Print and shaded views of the part. All mm, measured from the part's lowest x, y and z. A direction names the side the tool comes from. Round coordinates to 2 decimals unless told otherwise and drop trailing zeros. Loops run counter-clockwise (first coordinate to the right, second up) from the corner with the lowest first, then second, coordinate; pieces in that order, holes last. Notation, with made-up numbers: (-4.5, -31.75) - (25.5, -31.75) arc R16 ccw to (25.5, -18.75) - close; hole circle Ø5 at (-34.5, 20). An arc over 180 degrees is marked (long way). Answer as a JSON object with one key per item and string values.
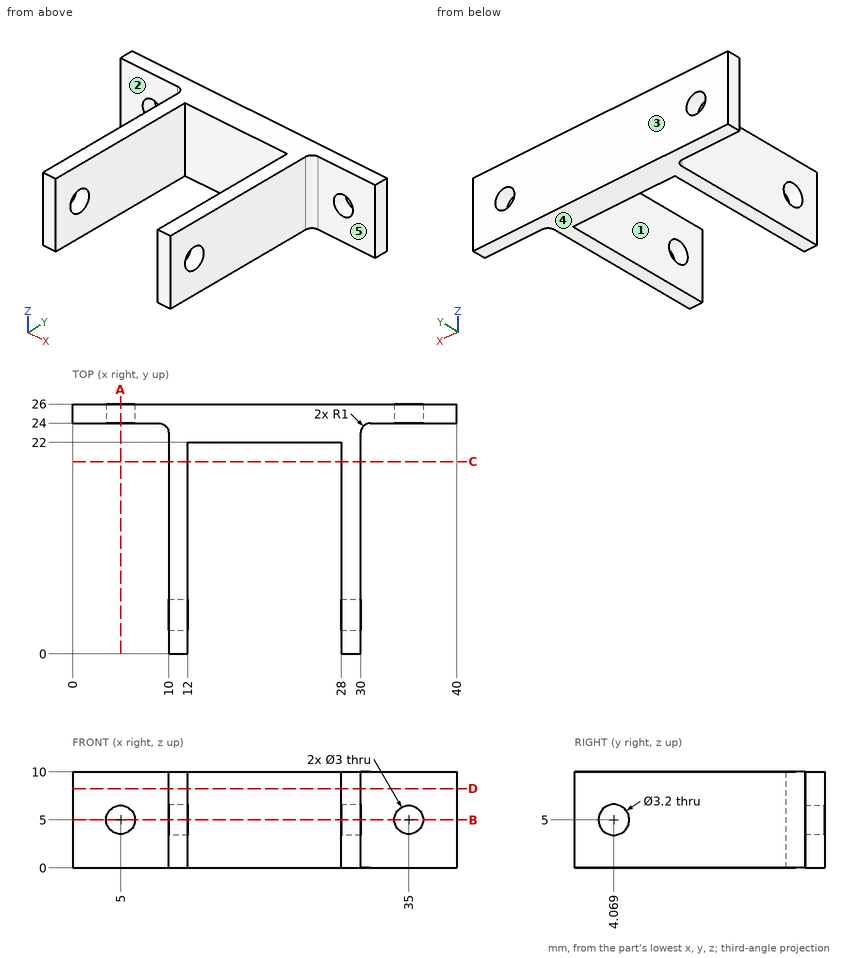
1) Slice it at A-A on x = 5. List the corners of the cut face in (y, z), then the cut area to 3 significant figures.
Values follow:
{"outline": "(24, 0) - (26, 0) - (26, 3.5) - (24, 3.5) - close; (24, 6.5) - (26, 6.5) - (26, 10) - (24, 10) - close", "area": "14.0 mm²"}
2) Slice it at C-C on y = 20. List the corners of the cut face in (x, z).
Values follow:
{"outline": "(10, 0) - (12, 0) - (12, 10) - (10, 10) - close; (28, 0) - (30, 0) - (30, 10) - (28, 10) - close"}
3) Slice it at D-D on z = 8.25. List the corners of the cut face in (x, y).
Values follow:
{"outline": "(0, 24) - (9, 24) arc R1 cw to (10, 23) - (10, 0) - (12, 0) - (12, 22) - (28, 22) - (28, 0) - (30, 0) - (30, 23) arc R1 cw to (31, 24) - (40, 24) - (40, 26) - (0, 26) - close"}
4) Slice it at B-B on z = 5. Count the separate pieces of the cut face and the enclosed holes in it.
Values follow:
{"separate pieces": "5", "enclosed holes": "0"}
5) Probe probe 1 along X at (y, z) = (24.5, 5); probe 2 along Z at (x, y) = (35, 24.85); probe 3 along Y at (x, z) = (29.1, 5). List the from-to ranges inside material, lowest first.
Values follow:
{"probe 1": "0 to 3.5, 6.5 to 33.5, 36.5 to 40", "probe 2": "0 to 3.5, 6.5 to 10", "probe 3": "0 to 2.47, 5.67 to 26"}
6) Tool access for the marked faces 1, 2, 3, 4 and 5: list every direction of +Z, -Z, +X, -X, +Y, -Y with a clear straight run to the whole face (end or side of a thin tool).
Values follow:
{"face 1": "+Z, -Z, -Y", "face 2": "+Z, -Z, -X, -Y", "face 3": "+Z, -Z, +X, -X, +Y", "face 4": "-Z, +X, -X, +Y, -Y", "face 5": "+Z, -Z, +X, -Y"}
7) Drop flat-ended pins along their axis: P1, Ø5, axis at x = 5, z = 5, coming from the -Y side; P2, Ø3, axis at y = 15.5, z = 5, coming from the +X side; P3, Ø2, axis at y = 20, z = 2, coming from the -X side. Give the stop position or say it passes through.
Values follow:
{"P1": "y = 24", "P2": "x = 30", "P3": "x = 10"}
